Input: dimensioned drawing with shaded views. Units: mm. Origin: part minimum x, y, z. A direction names the side the tool comes from. Round coordinates to 2 decimals unless told otherwise and drop trailing zeros. Write each loop counter-clockwise with the first axis right and the second up, starting at its lowest first coordinate (ties: lowest second). Pieces come first, ordered by that corner, then holes. Notation, with made-up numbers: M 70,2.5 L 117,2.5 A17 cw 117,21.5 Z; hole C -11,28 d8. An arc over 180 degrees is marked long. Answer in a Markdown table with one row per item. Add a question column.
Item 1: Cut plane D-D on z = 43.5. Return loops of the section in (x, y).
Item 2: Material intervals for probe 1 along X at (y, z) = (16.5, 34.5); probe 2 along Z at (x, y) = (4, 20.5); probe 3 along Z at (x, y) = (30, 26.5), sorted ascending.
Item 3: Set-up query: the marked faces 1 and 2. Return all of +Z, -Z, +X, -X, +Y, -Y with unobstructed straight access to the full face (end or side cutting, diameter ignored); none if empty.
Item 4: Cut plane C-C on z = 105. Return loops of the section in (x, y), and give its area (3 significant figures).
Item 5: Contact query for flat-ended pins moving along their axis: pin 1 (6 mm diameter, centred on x = 13.5, z = 39, fed in from -Y); pin 2 (8 mm diameter, centred on y = 11, z = 22, fed in from +X); pin 3 (1.5 mm diameter, centred on y = 25, z = 61, fed in from +X). Output: stop coordinate, or through.
Item 6: Cut plane A-A on x = 17. Return loops of the section in (y, z).
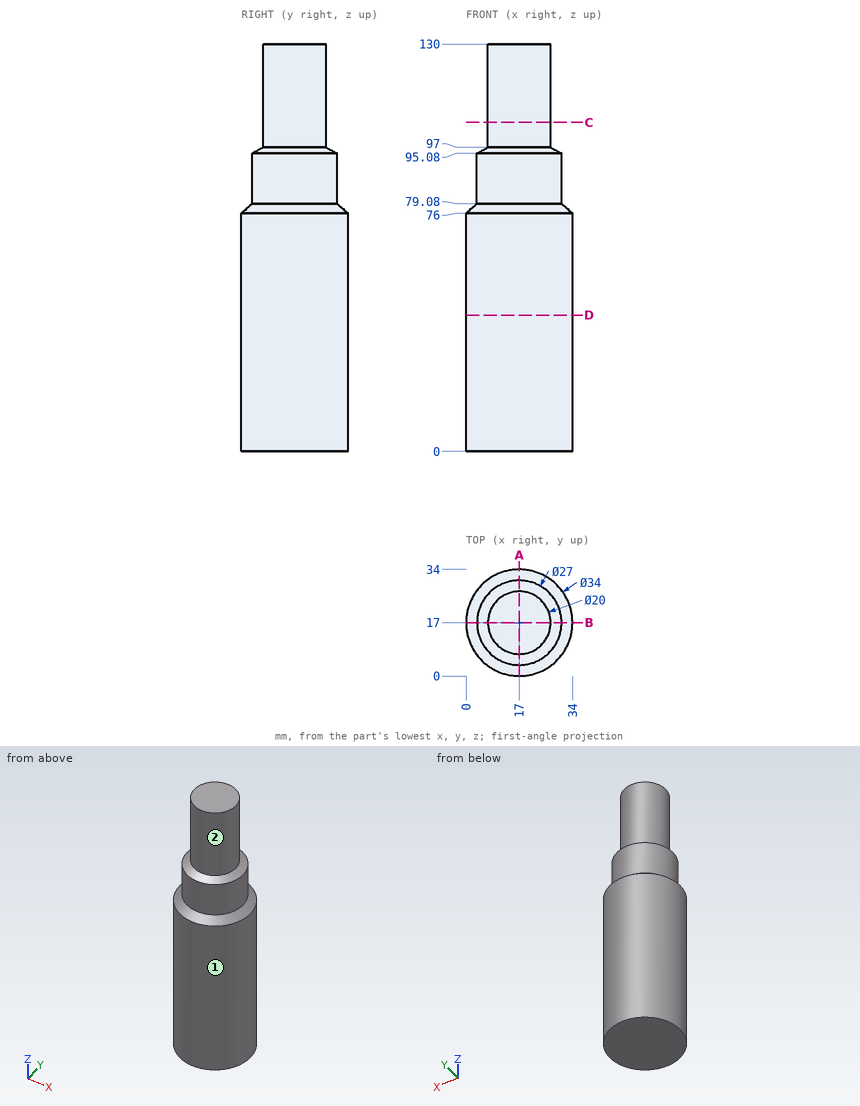
Results below:
| question | item | result |
|---|---|---|
| 1 | outline | C 17,17 d34 |
| 2 | probe 1 | 0.01 to 33.99 |
| 2 | probe 2 | 0 to 95.1 |
| 2 | probe 3 | 0 to 76.79 |
| 3 | face 1 | +Z, -Z |
| 3 | face 2 | +Z |
| 4 | outline | C 17,17 d20 |
| 4 | area | 314 mm2 |
| 5 | pin 1 | y = 0.01 |
| 5 | pin 2 | x = 33.88 |
| 5 | pin 3 | x = 32.38 |
| 6 | outline | M 0,0 L 34,0 L 34,76 L 30.5,79.08 L 30.5,95.08 L 27,97 L 27,130 L 7,130 L 7,97 L 3.5,95.08 L 3.5,79.08 L 0,76 Z |
